For this review, take the finished solid that the model builds, in its own axes (mm). A direction names the side the tool comes from. Coordinates: 2 decimals unless noted, no trailing zeros. Loops run counter-clockwise (first coordinate to the right, second up) from the corner with the lowest first, then second, coordinate; pieces in that order, holes last. Notation, with made-up numbers: M 41,10.5 L 49,10.5 A20 cw 49,48.5 Z; hole C -15.5,12 d5. An arc over 180 degrees is marked long. Answer as a JSON object with one key per item and string values. Group by question number.
Item 1: Wall thickness on L1, parallel to Y at x = 52.5, z = -17; L2, parallel to X at y = 23, z = -10: over which ranges is each line inside the solid? List them lowest first. Write a range as from..to.
Item 2: Add section D-D (z = -31). State the section outline as (x, y) points, then the cut area to 3 significant figures.
Item 3: Add section A-A (z = -13). State the section outline as (x, y) points.
Item 4: Add section C-C (x = 53). State the section outline as (y, z) points, then the cut area to 3 significant figures.
Item 5: Insertion check: pin 1 (8 mm diameter, centred on x = 31, z = -34, fed in from +Y); pin 2 (8 mm diameter, centred on y = 15.5, z = -35, fed in from +X); pin 3 (4 mm diameter, centred on y = 24, z = -33, fed in from +X). Each pin has a flat end and moves straight along its axis. Give the tip position at first contact, or say it passes through.
Item 6: Tool access review of faces 1 (the face through (23, 12, 0)), 2 (the face through (20, 20, -20)), 3 (the face through (45, 10, -20)): name each direction out of +Z, -Z, +X, -X, +Y, -Y from which nothing blocks a thin tool from reaching the whole face with its end or side.
Item 7: Add section B-B (y = 16). State the section outline as (x, z) points, then the cut area to 3 significant figures.
from build123d import *

# Parameters (mm, degrees)
SKETCH1_W           = 40
SKETCH1_H           = 10
BOSS_EXTRUDE2_DEPTH = 10
SKETCH1_4_W         = 40
SKETCH1_4_H         = 10
BOSS_EXTRUDE3_DEPTH = 60
BOSS_EXTRUDE4_DEPTH = 30


with BuildPart() as part:
    # Sketch1 → Boss-Extrude2 (new body)
    with BuildSketch(Plane(origin=(0, 0, 0), x_dir=(0, 0, -1), z_dir=(1, 0, 0))):
        Polygon((0, 30), (0, 10), (40, 10), align=None)
        Polygon((0, 30), (40, 10), (40, 30), align=None)
        with Locations((20, 5)):
            Rectangle(SKETCH1_W, SKETCH1_H)
    extrude(amount=BOSS_EXTRUDE2_DEPTH)

    # Sketch1_4 → Boss-Extrude3 (add)
    with BuildSketch(Plane(origin=(0, 0, 0), x_dir=(0, 0, -1), z_dir=(1, 0, 0))):
        with Locations((20, 5)):
            Rectangle(SKETCH1_4_W, SKETCH1_4_H)
    extrude(amount=BOSS_EXTRUDE3_DEPTH)

    # Sketch1_6 → Boss-Extrude4 (add)
    with BuildSketch(Plane(origin=(0, 0, 0), x_dir=(0, 0, -1), z_dir=(1, 0, 0))):
        Polygon((0, 30), (0, 10), (40, 10), align=None)
    extrude(amount=BOSS_EXTRUDE4_DEPTH)


solid = part.part
From the geometry:
{
 "1": {"L1": "y = 0..10", "L2": "x = 0..30"},
 "2": {"outline": "M 0,0 L 60,0 L 60,10 L 30,10 L 30,14.5 L 10,14.5 L 10,30 L 0,30 Z", "area": "890 mm²"},
 "3": {"outline": "M 0,0 L 60,0 L 60,10 L 30,10 L 30,23.5 L 10,23.5 L 10,30 L 0,30 Z"},
 "4": {"outline": "M 0,-40 L 10,-40 L 10,0 L 0,0 Z", "area": "400 mm²"},
 "5": {"pin 1": "stops at y = 14.94", "pin 2": "stops at x = 30", "pin 3": "stops at x = 10"},
 "6": {"face 1": "+Z, +X, -X, +Y, -Y", "face 2": "-Z, +X, +Y", "face 3": "+Z, -Z, +X, +Y"},
 "7": {"outline": "M 0,-40 L 10,-40 L 10,-28 L 30,-28 L 30,0 L 0,0 Z", "area": "960 mm²"}
}
